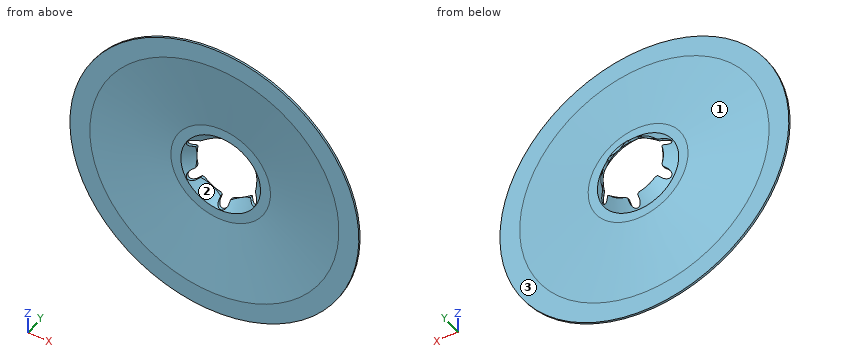
from build123d import *

# Parameters (mm, degrees)
CUT_EXTRUDE2_DEPTH = 10


with BuildPart() as part:
    # Sketch1 → Revolve1 (revolve)
    with BuildSketch(Plane(origin=(0, 0, 0), x_dir=(0, 0, -1), z_dir=(1, 0, 0))):
        Polygon((0, 0), (0, 0.2), (1.986725405, 0.2), (9.486725405, 1.2), (10.417157288, 1.2), (11.358578644, 2.141421356), (11.5, 2), (10.5, 1), (9.5, 1), (2, 0), align=None)
    revolve(axis=Axis((0, 1.2, -14.5), (0, -1, 0)))

    # Sketch3 → Cut-Extrude2 (cut)
    with BuildSketch(Plane(origin=(0, 0, 0), x_dir=(1, 0, 0), z_dir=(0, 1, 0))):
        with BuildLine():
            Line((3.25, 13.200961894), (3, 13.345299462))
            Line((3, 13.345299462), (3, 15.654700538))
            Line((3, 15.654700538), (3.25, 15.799038106))
            ThreePointArc((3.25, 15.799038106), (3.433012702, 16.482050808), (2.75, 16.665063509))
            Line((2.75, 16.665063509), (2.5, 16.520725942))
            Line((2.5, 16.520725942), (0.5, 17.675426481))
            Line((0.5, 17.675426481), (0.5, 17.964101615))
            ThreePointArc((0.5, 17.964101615), (0, 18.464101615), (-0.5, 17.964101615))
            Line((-0.5, 17.964101615), (-0.5, 17.675426481))
            Line((-0.5, 17.675426481), (-2.5, 16.520725942))
            Line((-2.5, 16.520725942), (-2.75, 16.665063509))
            ThreePointArc((-2.75, 16.665063509), (-3.433012702, 16.482050808), (-3.25, 15.799038106))
            Line((-3.25, 15.799038106), (-3, 15.654700538))
            Line((-3, 15.654700538), (-3, 13.345299462))
            Line((-3, 13.345299462), (-3.25, 13.200961894))
            ThreePointArc((-3.25, 13.200961894), (-3.433012702, 12.517949192), (-2.75, 12.334936491))
            Line((-2.75, 12.334936491), (-2.5, 12.479274058))
            Line((-2.5, 12.479274058), (-0.5, 11.324573519))
            Line((-0.5, 11.324573519), (-0.5, 11.035898385))
            ThreePointArc((-0.5, 11.035898385), (0, 10.535898385), (0.5, 11.035898385))
            Line((0.5, 11.035898385), (0.5, 11.324573519))
            Line((0.5, 11.324573519), (2.5, 12.479274058))
            Line((2.5, 12.479274058), (2.75, 12.334936491))
            ThreePointArc((2.75, 12.334936491), (3.433012702, 12.517949192), (3.25, 13.200961894))
        make_face()
    extrude(amount=CUT_EXTRUDE2_DEPTH, mode=Mode.SUBTRACT)


solid = part.part
Verification items for the finished model (mm, model axes). Face numbers are marked on the shaded views. Give positions to 0.01 mm unless a question says otherwise; leave off trailing zeros. Loops run counter-clockwise (first coordinate to the right, second up) from the corner with the lowest first, then second, coordinate; pieces in that order, holes last. Notation, with made-up numbers: (21.25, 21) - (66.25, 21) arc R28 cw to (66.25, 53) - close; hole circle Ø10 at (71, 83). An arc over 180 degrees is marked (long way). Write item = value, one per line. Start each with the question number.
Q1. Thickness scan on line 1 (Y direction, x = -12.5, z = -21); line 2 (X direction, y = 1.6, z = -17); line 3 (Y direction, x = 5.75, z = -4.5). Record the ranges inside material, lowest first.
Q2. Cross-section at A-A, the plane x = 0. Enter the section's corners in (y, z).
Q3. Mould release check, pull along Z, two halves, no side actions. Record for the marked faces 1, 2 and 3: released by +Z, released by -Z, zero draft, split by the parting line, or undercut.
Q4. Cross-section at B-B, the plane y = 0.65. Enter the section's corners in (x, z) (3 decimals).
Q5. Depth check by flat-ended pin: P1, Ø6, axis at x = 9.5, z = -4.5, coming from the +Y side; P2, Ø11, axis at x = 1.5, z = -14, coming from the -Y side; P3, Ø1.5, axis at x = -8.5, z = -14, coming from the -Y side. Enter the tip coordinate at first touch or a pass-through.
Answer key:
q1.line_1 = 0 to 0.2
q1.line_2 = -2.7 to -2.3, 2.3 to 2.7
q1.line_3 = 0.13 to 0.33
q2.outline = (0, -29) - (0.2, -29) - (0.2, -27.01) - (1.2, -19.51) - (1.2, -18.58) - (1.32, -18.46) - (1.04, -18.46) - (1, -18.5) - (1, -19.5) - (0, -27) - close; (0, -2) - (1, -9.5) - (1, -10.5) - (1.04, -10.54) - (1.32, -10.54) - (1.2, -10.42) - (1.2, -9.49) - (0.2, -1.99) - (0.2, 0) - (0, 0) - close
q3.face_1 = split by the parting line
q3.face_2 = undercut
q3.face_3 = zero draft
q4.outline = circle Ø18.277 at (0, -14.5); hole circle Ø15.25 at (0, -14.5)
q5.P1 = 0.43
q5.P2 = 0.72
q5.P3 = 0.43
